The model under review builds one solid part; all positions refer to its coordinate system, in mm. A direction names the side the tool comes from. Coordinates: 2 decimals unless noted, no trailing zeros. Write each loop counter-clockwise with the first axis right and the second up, starting at its lowest first coordinate (ties: lowest second). Pieces come first, ordered by that corner, then holes. Notation, with made-up numbers: (12, 45) - (21, 45) arc R26 cw to (21, 61) - close; hole circle Ø11 at (-34, 60.5). An arc over 180 degrees is marked (long way). Put each result on its own line as item: value. Start each with the question number.
Item 1: Consider section A-A on y = -4.25. Give the boundary of the cut face in (x, z), then the cut area to 3 significant figures.
Item 2: Machinability: for faces 1 (the face through (-3.483, 3.427, 9.86)), 2 (the face through (3.5, 3.46, 9.86)), 3 (the face through (-2.207, 4.395, 9.86)), which of the approach directions +Z, -Z, +X, -X, +Y, -Y give a long, thin tool a straight path to every point of the face, cutting with its end or side? Answer none if there is none.
Item 3: Consider section C-C on y = -3. Give the boundary of the cut face in (x, z).
Item 4: To check wall thickness, follow L1, parallel to X at y = -3.75, z = 3.5; L2, parallel to X at y = 5, z = 3.5; L3, parallel to Y at x = 3.5, z = 14.5. State the ranges of each line that lie inside material, in increasing order. Write a range as [from, to].
Item 5: For pin 1 (1 mm diameter, centred on x = 1.5, z = 3.5, fed in from +Y); pin 2 (2 mm diameter, centred on y = 3.5, z = 6, fed in from -X), all flat-tipped, find the tip position at first contact; note any pin that passes through.
Item 6: Mouldability with a two-part tool opening along X and no side actions: class faces 4 (the face through (-0.8, -4.85, 9.86)), 5 (the face through (0, -6, 10)), 6 (the face through (-2.18, -4.37, 9.86)), 7 (the face through (3.483, -3.427, 9.86)) as pulls with the +X half, pulls with the -X half, needs draft (parallel to the pull), parting line crosses it, or undercut.
Item 7: Consider section B-B on x = 4.75. Give the boundary of the cut face in (y, z).
Autodesk Inventor part; units mm, degrees
ref_plane "Work Plane2" through (0, 0, 10) normal (0, 0, 1) x (1, 0, 0)
ref_plane "Work Plane8" through (0, 0, 0) normal (0.9510565, 0.309017, 0) x (0, 0, 1)
ref_plane "Work Plane9" through (0, 0, 0) normal (1, 0, 0) x (0, 1, 0)
sketch "Sketch1" plane through (0, 0, 0) normal (0, 0, 1) x (1, 0, 0)
  circle A0 centre (0, 0) radius 6
  dimension "d0" = 12
extrude "Extrusion1" add sketch "Sketch1" along normal blind 20
ref_plane "Work Plane2" through (0, 0, 10) normal (0, 0, 1) x (1, 0, 0)
sketch "Sketch2" plane through (0, 0, 0) normal (0, 0, -1) x (-1, 0, 0)
  circle A0 centre (0, 0) radius 6
  circle A1 centre (0, 0) radius 5
  dimension "d3" = 10
surface extrude "Pitch Diameter" sketch "Sketch2" against normal through all shown no curves A1
ref_plane "Work Plane8" through (0, 0, 0) normal (0.9510565, 0.309017, 0) x (0, 0, 1)
ref_plane "Work Plane9" through (0, 0, 0) normal (1, 0, 0) x (0, 1, 0)
spur gear teeth "Spur Gear" teeth 10 pitch diameter 10 tip diameter 12 root diameter 7.5 face width 20 start plane through (0, 0, 0) normal (0, 0, -1) x (-1, 0, 0)
equation "\"d0\" = da_da"
equation "\"d1\" = da_b"
equation "\"d3\" = da_d"
equation "\"d16\" = da_aw"
equation "\"d43\" = da_aw"
equation "\"d46\" = da_aw"
properties part number "Spur Gear1" material "Steel"
Report:
1. outline: (-3.81, 0) - (-2.06, 0) - (-2.06, 20) - (-3.81, 20) - close; (-0.87, 0) - (0.87, 0) - (0.87, 20) - (-0.87, 20) - close; (2.06, 0) - (3.81, 0) - (3.81, 20) - (2.06, 20) - close
1. area: 105 mm²
2. face 1: +Z, -Z, -X
2. face 2: +Z, -Z, +X
2. face 3: +Z, -Z, +Y
3. outline: (-3.25, 0) - (3.25, 0) - (3.25, 20) - (-3.25, 20) - close
4. L1: [-3.63, -1.64], [-0.88, 0.88], [1.64, 3.63]
4. L2: [-3.32, -2.96], [-0.77, 0.77], [2.96, 3.32]
4. L3: [-4.87, -3.46], [-2.06, 2.06], [3.46, 4.87]
5. pin 1: y = 4.18
5. pin 2: x = -3.88
6. face 4: undercut
6. face 5: parting line crosses it
6. face 6: undercut
6. face 7: pulls with the +X half
7. outline: (-2.3, 0) - (-0.68, 0) - (-0.68, 20) - (-2.3, 20) - close; (0.68, 0) - (2.3, 0) - (2.3, 20) - (0.68, 20) - close
